```python
from build123d import *

# Parameters (mm, degrees)
F_70X45X5_1_DEPTH   = 2040
CUT_EXTRUDE_1_REACH = 2062.951
SKETCH_12_R         = 7
CUT_EXTRUDE_2_REACH = 2062.951
SKETCH_13_R         = 7
CHAMFER_1_SIZE      = 30
CHAMFER_2_SIZE      = 30


with BuildPart() as part:
    # 草图11 → 不等边角钢 70X45X5(1) (new body)
    with BuildSketch(Plane(origin=(1020, 1766.69182372, 0), x_dir=(0.86602540378444, -0.49999999999999784, 0), z_dir=(-0.49999999999999784, -0.86602540378444, 0))):
        with BuildLine():
            Line((0, 70), (0, 0))
            Line((0, 0), (45, 0))
            Line((45, 0), (45, 3.33))
            ThreePointArc((45, 3.33), (44.510868325, 4.510868325), (43.33, 5))
            Line((43.33, 5), (12.5, 5))
            ThreePointArc((12.5, 5), (7.196699141, 7.196699141), (5, 12.5))
            Line((5, 12.5), (5, 68.33))
            ThreePointArc((5, 68.33), (4.510868325, 69.510868325), (3.33, 70))
            Line((3.33, 70), (0, 70))
        make_face()
    extrude(amount=F_70X45X5_1_DEPTH)

    # 草图12 → 切除-拉伸1 (cut, up to next)
    with BuildSketch(Plane(origin=(0, 0, 0), x_dir=(0, 0, 1), z_dir=(-0.86602540378444, 0.49999999999999784, 0)), mode=Mode.PRIVATE) as cut_extrude_1_sk1:
        with Locations(Location((40, 30, 0), (0, 0, 270))):
            Circle(SKETCH_12_R)
    cut_extrude_1_tool1 = extrude(cut_extrude_1_sk1.sketch, amount=-CUT_EXTRUDE_1_REACH, mode=Mode.PRIVATE) & part.part
    # 草图12 → 切除-拉伸1 (cut, up to next)
    with BuildSketch(Plane(origin=(0, 0, 0), x_dir=(0, 0, 1), z_dir=(-0.86602540378444, 0.49999999999999784, 0)), mode=Mode.PRIVATE) as cut_extrude_1_sk2:
        with Locations(Location((40, 110, 0), (0, 0, 270))):
            Circle(SKETCH_12_R)
    cut_extrude_1_tool2 = extrude(cut_extrude_1_sk2.sketch, amount=-CUT_EXTRUDE_1_REACH, mode=Mode.PRIVATE) & part.part
    add(cut_extrude_1_tool1.solids().sort_by_distance((15, 25.980762, 40))[0], mode=Mode.SUBTRACT)
    add(cut_extrude_1_tool2.solids().sort_by_distance((55, 95.262794, 40))[0], mode=Mode.SUBTRACT)

    # 草图13 → 切除-拉伸2 (cut, up to next)
    with BuildSketch(Plane(origin=(0, 0, 0), x_dir=(0, 0, 1), z_dir=(-0.86602540378444, 0.49999999999999784, 0)), mode=Mode.PRIVATE) as cut_extrude_2_sk1:
        with Locations(Location((40.004723234, 1930, 0), (0, 0, 270))):
            Circle(SKETCH_13_R)
    cut_extrude_2_tool1 = extrude(cut_extrude_2_sk1.sketch, amount=-CUT_EXTRUDE_2_REACH, mode=Mode.PRIVATE) & part.part
    # 草图13 → 切除-拉伸2 (cut, up to next)
    with BuildSketch(Plane(origin=(0, 0, 0), x_dir=(0, 0, 1), z_dir=(-0.86602540378444, 0.49999999999999784, 0)), mode=Mode.PRIVATE) as cut_extrude_2_sk2:
        with Locations(Location((40.004723234, 2010, 0), (0, 0, 270))):
            Circle(SKETCH_13_R)
    cut_extrude_2_tool2 = extrude(cut_extrude_2_sk2.sketch, amount=-CUT_EXTRUDE_2_REACH, mode=Mode.PRIVATE) & part.part
    add(cut_extrude_2_tool1.solids().sort_by_distance((965, 1671.429029, 40.004723))[0], mode=Mode.SUBTRACT)
    add(cut_extrude_2_tool2.solids().sort_by_distance((1005, 1740.711062, 40.004723))[0], mode=Mode.SUBTRACT)

    # 倒角1
    # the kernel refuses this chamfer: 30 mm, written as the material it takes off along each edge
    with BuildSketch(Plane(origin=(1089.698148536, 1726.451578901, 70), x_dir=(-0.49981095845564616, -0.8656979742248816, 0.027495876610586854), z_dir=(-0.86602540378444, 0.49999999999999784, 0))) as chamfer_1_piece_1:
        Polygon((CHAMFER_1_SIZE * 0.999621916911, -CHAMFER_1_SIZE * 0.0274958766106), (-CHAMFER_1_SIZE * 0.0274958766106, -CHAMFER_1_SIZE * 0.999621916911), (0, 0), align=None)
    extrude(amount=157.630979278, mode=Mode.SUBTRACT)

    # 倒角2
    # the kernel refuses this chamfer: 30 mm, written as the material it takes off along each edge
    with BuildSketch(Plane(origin=(69.698148536, -40.240244819, 70), x_dir=(-0.013747938305293054, -0.023812127644090075, -0.9996219169112966), z_dir=(-0.86602540378444, 0.49999999999999784, 0))) as chamfer_2_piece_1:
        Polygon((CHAMFER_2_SIZE * 0.999621916911, -CHAMFER_2_SIZE * 0.0274958766106), (-CHAMFER_2_SIZE * 0.0274958766106, -CHAMFER_2_SIZE * 0.999621916911), (0, 0), align=None)
    extrude(amount=157.630979278, mode=Mode.SUBTRACT)


solid = part.part
```
For this review, take the finished solid that the model builds, in its own axes (mm). A direction names the side the tool comes from. Coordinates: 2 decimals unless noted, no trailing zeros. Answer as a JSON object with one key per item and string values. Group by question number.
1. Clearance check with flat-ended pins moving along their axes: P1, Ø6, axis at x = 203, z = 48, coming from the -Y side; P2, Ø1, axis at y = 1443, z = 34.5, coming from the -X side; P3, Ø8, axis at x = 404, z = 60, coming from the +Y side. State where each tip first meets the part, or that it passes through.
2. For faces 1 (the flat face through (521.47, 893.21, 40.02)), 2 (the flat face through (7.85, -4.53, 5.28)), list the 3-axis set-ups (+Z, -Z, +X, -X, +Y, -Y) from which the entire face can be reached by the end or side of a thin tool; tool diameter is ignored.
3. For probe 1 along X at (y, z) = (1177, 16.5); probe 2 along Y at (x, z) = (435, 33); probe 3 along X at (y, z) = (1534, 12), list the stretches that pass through material, from the lowest coordinate up.
Final values:
{
 "1": {"P1": "y = 336.41", "P2": "x = 832.83", "P3": "y = 706.68"},
 "2": {"face 1": "+Z, +X, -Y", "face 2": "+Z, -Z, -X, -Y"},
 "3": {"probe 1": "679.54 to 685.31", "probe 2": "743.44 to 753.44", "probe 3": "885.66 to 891.45"}
}
